Read the model definition and answer for the solid it produces. Units are mm, in the model's axes. Give positions to 0.01 mm unless a question says otherwise; leave off trailing zeros. Order: outer loops, then holes, each group sorted by start corner. A loop starts at its lowest first (then second) coordinate and runs counter-clockwise, first axis right, second up.
```python
from build123d import *

# Parameters (mm, degrees)
EXTRUDE_THIN1_DEPTH = 12.5


with BuildPart() as part:
    # Sketch1 → Extrude-Thin1 (new, symmetric)
    with BuildSketch(Plane.XY):
        with BuildLine():
            Line((252.626703921, -22.113309703), (24.803089564, 64.923468392))
            ThreePointArc((24.803089564, 64.923468392), (-68.346291243, 12.610887097), (0, -69.5))
            Line((0, -69.5), (243.883168751, -69.5))
            ThreePointArc((243.883168751, -69.5), (267.976465664, -49.445564516), (252.626703921, -22.113309703))
        make_face()
        with BuildLine():
            Line((251.912945948, -23.981610952), (24.089331591, 63.055167144))
            ThreePointArc((24.089331591, 63.055167144), (-66.379491495, 12.247983871), (0, -67.5))
            Line((0, -67.5), (243.883168751, -67.5))
            ThreePointArc((243.883168751, -67.5), (266.009665916, -49.08266129), (251.912945948, -23.981610952))
        make_face(mode=Mode.SUBTRACT)
    extrude(amount=EXTRUDE_THIN1_DEPTH, both=True)

    # Sweep1: sweep along a path in Sketch1<3>
    with BuildLine(Plane.XY) as sweep1_path:
        Line((0, -67.5), (243.883168751, -67.5))
        ThreePointArc((243.883168751, -67.5), (266.009665916, -49.08266129), (251.912945948, -23.981610952))
        Line((251.912945948, -23.981610952), (24.089331591, 63.055167144))
        ThreePointArc((24.089331591, 63.055167144), (-66.379491495, 12.247983871), (0, -67.5))
    # Sketch2 → Sweep1 (sweep)
    with BuildSketch(Plane(origin=(0, 0, 0), x_dir=(0, 0, -1), z_dir=(1, 0, 0))):
        Polygon((-3, -67.5), (-2, -62.5), (2, -62.5), (3, -67.5), align=None)
    sweep(path=sweep1_path.line)


solid = part.part
```
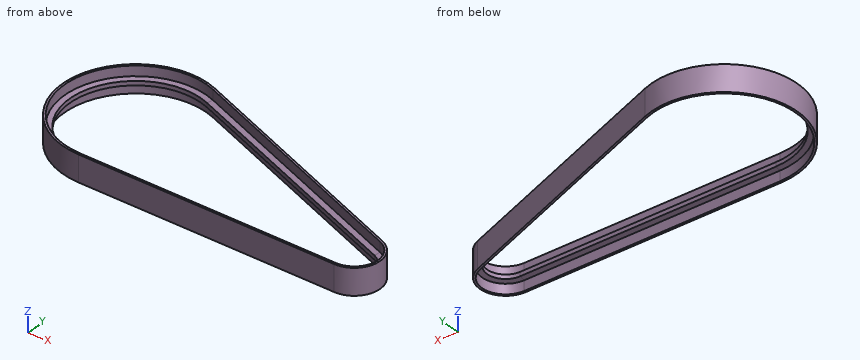
1) The part is cut by section C-C on x = 34.5. Determine the outline of the cut face in (y, z).
Final values:
outline: (-69.5, -12.5) - (-67.5, -12.5) - (-67.5, -3) - (-62.5, -2) - (-62.5, 2) - (-67.5, 3) - (-67.5, 12.5) - (-69.5, 12.5) - close; (53.73, -2) - (59.08, -3) - (59.08, -12.5) - (61.22, -12.5) - (61.22, 12.5) - (59.08, 12.5) - (59.08, 3) - (53.73, 2) - close
2) Given pin 1 (10.5 mm diameter, centred on x = 94.5, z = 8, fed in from +Y); pin 2 (1 mm diameter, centred on y = 16, z = 9, fed in from -X); pin 3 (10.5 mm diameter, centred on x = 84, z = -10, fed in from +Y), each flat-ended and moving along its own axis, determine where each tip first touches the part or whether it passes through.
Final values:
pin 1: stops at y = 40.3
pin 2: stops at x = -67.75
pin 3: stops at y = 44.31
3) The part is cut by section A-A on z = -7.75. Determine the outline of the cut face in (x, y).
Final values:
outline: (0, -69.5) - (243.88, -69.5) arc R24.5 ccw to (252.63, -22.11) - (24.8, 64.92) arc R69.5 ccw (long way) to start; hole (0, -67.5) - (243.88, -67.5) arc R22.5 ccw to (251.91, -23.98) - (24.09, 63.06) arc R67.5 ccw (long way) to start
4) The part is cut by section B-B on y = 0. Determine the outline of the cut face in (x, z), and give its area (3 significant figures).
Final values:
outline: (-69.5, -12.5) - (-67.5, -12.5) - (-67.5, -3) - (-62.5, -2) - (-62.5, 2) - (-67.5, 3) - (-67.5, 12.5) - (-69.5, 12.5) - close; (175.13, -2) - (189.14, -3) - (189.14, -12.5) - (194.74, -12.5) - (194.74, 12.5) - (189.14, 12.5) - (189.14, 3) - (175.13, 2) - close
area: 285 mm2
5) Consider L1, parallel to Y at x = 0, z = -5.5; L2, parallel to Y at x = 55.5, z = -9; L3, parallel to X at y = -53, z = -9. Determine where each line is inside the solid, lowest interval first.
Final values:
L1: y = -69.5 to -67.5, 67.5 to 69.5
L2: y = -69.5 to -67.5, 51.06 to 53.2
L3: x = -44.96 to -41.8, 264.91 to 267.04
